```python
from build123d import *

# Parameters (mm, degrees)
SKETCH1_W              = 30
SKETCH1_H              = 25
BASE_FLANGE1_DEPTH     = 3
SKETCHED_START         = -15
SKETCHED_BEND1_DEPTH   = 30
SKETCHED_BEND1_2_DEPTH = 30


# Read off the part's stored shape, not the designer's step: Sketched Bend1
# Sheet-metal steps are written as plain solids
with BuildPart() as part:
    # Sketch1 → Base-Flange1 (new body)
    with BuildSketch(Plane.XY):
        Rectangle(SKETCH1_W, SKETCH1_H)
    extrude(amount=-BASE_FLANGE1_DEPTH)

    # Sketched Bend1 outline → Sketched Bend1 (cut)
    with BuildSketch(Plane.YZ.offset(SKETCHED_START)):
        with BuildLine():
            Line((12.5, 0), (1.661860688, 0))
            ThreePointArc((1.661860688, 0), (-0.534291735, -2.196152423), (-3.534291735, -3))
            Line((-3.534291735, -3), (12.5, -3))
            Line((12.5, -3), (12.5, 0))
        make_face()
    extrude(amount=SKETCHED_BEND1_DEPTH, mode=Mode.SUBTRACT)

    # Sketched Bend1 2 outline → Sketched Bend1 2 (add)
    with BuildSketch(Plane.YZ.offset(SKETCHED_START)):
        with BuildLine():
            Line((2.465708265, 3), (2.465708265, 11.965708265))
            Line((2.465708265, 11.965708265), (-0.534291735, 11.965708265))
            Line((-0.534291735, 11.965708265), (-0.534291735, 3))
            ThreePointArc((-0.534291735, 3), (-1.412971392, 0.878679657), (-3.534291735, 0))
            Line((-3.534291735, 0), (1.661860688, 0))
            ThreePointArc((1.661860688, 0), (2.261263223, 1.447085729), (2.465708265, 3))
        make_face()
    extrude(amount=SKETCHED_BEND1_2_DEPTH)


solid = part.part
```
Could you check a few things on this model? Use its own coordinates, in mm. A direction names the side the tool comes from. Round coordinates to 2 decimals unless told otherwise and drop trailing zeros. Loops run counter-clockwise (first coordinate to the right, second up) from the corner with the lowest first, then second, coordinate; pieces in that order, holes last.
Q1. Please list where these lines run through material, in increasing order: L1, parallel to Y at x = 7, z = 7.75; L2, parallel to Z at x = -0.75, y = -4.25; L3, parallel to Z at x = -8, y = -2.
Q2. For P1, Ø6, axis at y = -4, z = 8.5, coming from the +X side; P2, Ø8, axis at x = -5, z = -0.5, coming from the +Y side; P3, Ø4.5, axis at x = 4.5, y = -6, coming from the +Z side, each with a flat end and sliding along its axis, tell me the tip position at first contact or that it passes through.
Q3. I want a section at A-A (x = -2.75). Write out the boundary of the cut face in (y, z), and give its area (3 significant figures).
Q4. I want a section at C-C (y = -4.5). Write out the boundary of the cut face in (x, z), and give its area (3 significant figures).
Q5. I want a section at B-B (z = 9). Write out the boundary of the cut face in (x, y), and give its area (3 significant figures).
Q6. On a 3-axis mill with a long thin cutter (end or side, diameter ignored), from which of +Z, -Z, +X, -X, +Y, -Y can I reach the whole of each face in a straight line? I mean faces 1 (the flat face through (0, -0.534, 8)), 2 (the flat face through (0, -12.5, -1)). Say none if no direction works.
Answer below:
1. L1: y = -0.53 to 2.47
1. L2: z = -3 to 0
1. L3: z = -2.8 to 0.42
2. P1: passes through
2. P2: stops at y = 2.47
2. P3: stops at z = 0
3. outline: (-12.5, -3) - (-3.53, -3) arc R6 ccw to (2.47, 3) - (2.47, 11.97) - (-0.53, 11.97) - (-0.53, 3) arc R3 cw to (-3.53, 0) - (-12.5, 0) - close
3. area: 75.0 mm2
4. outline: (-15, -3) - (15, -3) - (15, 0) - (-15, 0) - close
4. area: 90.0 mm2
5. outline: (-15, -0.53) - (15, -0.53) - (15, 2.47) - (-15, 2.47) - close
5. area: 90.0 mm2
6. face 1: +Z, +X, -X, -Y
6. face 2: +Z, -Z, +X, -X, -Y
